from build123d import *

# Parameters (mm, degrees)
BOSS_EXTRUDE1_DEPTH = 6
SKETCH2_W           = 6
SKETCH2_H           = 3.9
BOSS_EXTRUDE2_DEPTH = 8
SKETCH3_R           = 2
CUT_EXTRUDE2_DEPTH  = 24.194962869
FILLET1_R           = 2
SKETCH6_W           = 5.996508816
SKETCH6_H           = 4.3
BOSS_EXTRUDE4_DEPTH = 6
SKETCH7_R           = 1.5
CUT_EXTRUDE3_DEPTH  = 26.803718238


with BuildPart() as part:
    # Sketch1 → Boss-Extrude1 (new body)
    with BuildSketch(Plane.XY):
        Polygon((-31.610053316, -13.34695045), (-31.610053316, -34.17695045), (-31.610053316, -42.01579246), (-25.132618973, -44.373385755), (-20.693197512, -32.176175537), (-26.049445451, -30.226660721), (-22.400090521, -20.200140457), (-17.043842583, -22.149655274), (-15.333741866, -17.45119217), (-26.610053316, -13.34695045), align=None)
    extrude(amount=BOSS_EXTRUDE1_DEPTH)

    # Sketch2 → Boss-Extrude2 (add)
    with BuildSketch(Plane.ZY.offset(31.610053316)):
        with Locations((3, -23.128422886)):
            Rectangle(SKETCH2_W, SKETCH2_H)
    extrude(amount=BOSS_EXTRUDE2_DEPTH)

    # Sketch3 → Cut-Extrude2 (cut, through all)
    with BuildSketch(Plane(origin=(0, -21.178422886, 0), x_dir=(1, 0, 0), z_dir=(0, 1, 0))):
        with Locations((-36.339467267, -3)):
            Circle(SKETCH3_R)
    extrude(amount=-CUT_EXTRUDE2_DEPTH, mode=Mode.SUBTRACT)

    # Fillet1
    fillet1_edges = [part.edges().sort_by_distance(p)[0] for p in [
        (-39.610053316, -23.128422886, 0),
        (-39.610053316, -23.128422886, 6),
    ]]
    fillet(fillet1_edges, radius=FILLET1_R)

    # Sketch6 → Boss-Extrude4 (add)
    with BuildSketch(Plane.XY.offset(6)):
        with Locations((-27.594946536, -37.000668688)):
            Rectangle(SKETCH6_W, SKETCH6_H)
    extrude(amount=BOSS_EXTRUDE4_DEPTH)

    # Sketch7 → Cut-Extrude3 (cut, through all)
    with BuildSketch(Plane.XZ.offset(39.150668688)):
        with Locations((-27.594946536, 9)):
            Circle(SKETCH7_R)
    extrude(amount=-CUT_EXTRUDE3_DEPTH, mode=Mode.SUBTRACT)


solid = part.part
Build history of the part. All positions in model axes, mm. A direction names the side the tool comes from. Round coordinates to 2 decimals unless told otherwise and drop trailing zeros. Write each loop counter-clockwise with the first axis right and the second up, starting at its lowest first coordinate (ties: lowest second). Pieces come first, ordered by that corner, then holes. Notation, with made-up numbers: (62, -20) -> (70, -20) arc R11 ccw to (70, -12) -> close; hole circle Ø8 at (40, 74). An arc over 180 degrees is marked (long way). Write item = value, one per line.
(1) Band-saw the part on B-B (x = -36.75). Give the cut face in (y, z).
Answer:
outline = (-25.08, 0) -> (-21.18, 0) -> (-21.18, 1.04) -> (-25.08, 1.04) -> close; (-25.08, 4.96) -> (-21.18, 4.96) -> (-21.18, 6) -> (-25.08, 6) -> close
(2) Flat gauge pins, fed straight in: pin 1 (6 mm diameter, centred on y = -21, z = 1.5, fed in from +X); pin 2 (4.5 mm diameter, centred on y = -37, z = 8.5, fed in from +X); pin 3 (6.5 mm diameter, centred on x = -36, z = 1.5, fed in from -Y). Where does each tip first touch, or does it go through?
Answer:
pin_1 = -15.53
pin_2 = -24.6
pin_3 = -25.08
(3) Tool access for faces 5 (the face through (-30.593, -37, 9)), 6 (the face through (-31.61, -33, 3)), 7 (the face through (-24.597, -37, 9)), 8 (the face through (-29, -34.851, 8)): list every direction of +Z, -Z, +X, -X, +Y, -Y with a clear straight run to the whole face (end or side of a thin tool).
Answer:
face_5 = +Z, -X, +Y, -Y
face_6 = +Z, -Z, -X, -Y
face_7 = +Z, +X, +Y, -Y
face_8 = +Z, +X, -X, +Y
(4) Two-plate mould, pull along X, no slides. Class faces 1 (the face through (-24.25, -25.28, 2.96)), 2 (the face through (-29, -13.347, 3)), 3 (the face through (-39.61, -23, 3)), 4 (the face through (-27.92, -37.031, 7.536)): pulls with the +X half, pulls with the -X half, needs draft (parallel to the pull), parting line crosses it, or undercut.
Answer:
face_1 = undercut
face_2 = needs draft
face_3 = pulls with the -X half
face_4 = undercut
(5) Band-saw the part on A-A (z = 3). Give the cut face in (x, y).
Answer:
outline = (-39.61, -25.08) -> (-38.34, -25.08) -> (-38.34, -21.18) -> (-39.61, -21.18) -> close; (-34.34, -25.08) -> (-31.61, -25.08) -> (-31.61, -42.02) -> (-25.13, -44.37) -> (-20.69, -32.18) -> (-26.05, -30.23) -> (-22.4, -20.2) -> (-17.04, -22.15) -> (-15.33, -17.45) -> (-26.61, -13.35) -> (-31.61, -13.35) -> (-31.61, -21.18) -> (-34.34, -21.18) -> close
(6) Probe L1, parallel to Z at x = -31, y = -24.5; L2, parallel to Y at x = -29, z = 11; L3, parallel to Z at x = -26.25, y = -37. List the from-to ranges inside material, lowest first.
Answer:
L1 = 0 to 6
L2 = -39.15 to -34.85
L3 = 0 to 8.34, 9.66 to 12
(7) Band-saw the part on D-D (x = -33). Give the cut face in (y, z).
Answer:
outline = (-25.08, 0) -> (-21.18, 0) -> (-21.18, 6) -> (-25.08, 6) -> close
(8) Band-saw the part on C-C (z = 9). Give the cut face in (x, y).
Answer:
outline = (-30.59, -39.15) -> (-29.09, -39.15) -> (-29.09, -34.85) -> (-30.59, -34.85) -> close; (-26.09, -39.15) -> (-24.6, -39.15) -> (-24.6, -34.85) -> (-26.09, -34.85) -> close
